Design review of the part built by this model. Coordinates are the model's own, in mm. A direction names the side the tool comes from. Give positions to 0.01 mm unless a question says otherwise; leave off trailing zeros. Loops run counter-clockwise (first coordinate to the right, second up) from the corner with the lowest first, then second, coordinate; pieces in that order, holes last. Notation, with made-up numbers: (-20.5, 74.25) -> (-9.5, 74.25) arc R20 cw to (-9.5, 101.25) -> close; hole circle Ø2 at (8.5, 58). An arc over 180 degrees is marked (long way). Use CSV: the item, a comma, the result in double quotes. Start each with the question number.
Item 1: We need section A-A (x = 6.5). State the section outline as (y, z) points.
Item 2: Clearance check with flat-ended pins moving along their axes: pin 1 (4.5 mm diameter, centred on x = 5, y = 23, fed in from +Z); pin 2 (1.7 mm diameter, centred on x = 6, y = 22.5, fed in from -Z); pin 3 (1 mm diameter, centred on x = 9.5, z = -1.5, fed in from +Y). State where each tip first meets the part, or that it passes through.
Item 3: The part is to be moulded in two halves that separate along Z. For faces 1 (the face through (5.4, 18.4, -1.8)), 2 (the face through (6, 18, -5.6)), 3 (the face through (9.24, 21.85, -2.43)), 4 (the face through (5, 23, -3.89)), say which applies: +Z half, -Z half, draft (parallel to the pull), parting line (faces both ways), or undercut.
Item 4: We need section C-C (z = -5.25). State the section outline as (x, y) points, plus the area to 3 significant figures.
Item 5: Wall thickness on line 1 along Z through (x, y) = (3.25, 6); line 2 along Z through (x, y) = (3.75, 3); line 3 along Z through (x, y) = (7.25, 22): over which ranges is each line inside the solid? List them lowest first. Write a range as from..to.
Item 6: For faces 5 (the face through (9.4, 17.89, -4.91)), 6 (the face through (5, 17.4, -6)), 7 (the face through (6, 5, -2.75)), list the 3-axis set-ups (+Z, -Z, +X, -X, +Y, -Y) from which the entire face can be reached by the end or side of a thin tool; tool diameter is ignored.
Item 7: We need section D-D (y = 24). State the section outline as (x, z) points (3 decimals), plus the area to 3 significant figures.
from build123d import *

# Parameters (mm, degrees)
BOSS_EXTRUDE1_DEPTH = 17.4
BOSS_EXTRUDE2_DEPTH = 1
BOSS_EXTRUDE3_DEPTH = 7
CUT_EXTRUDE1_DEPTH  = 4
CUT_EXTRUDE2_DEPTH  = 6.5
BOSS_EXTRUDE4_DEPTH = 2.1


with BuildPart() as part:
    # Sketch1 → Boss-Extrude1 (new body)
    with BuildSketch(Plane(origin=(0, 0, 0), x_dir=(1, 0, 0), z_dir=(0, 1, 0))):
        with BuildLine():
            Line((3.29, 0), (7.71, 0))
            ThreePointArc((7.71, 0), (10.03638131, 0.96361869), (11, 3.29))
            Line((11, 3.29), (11, 3.31))
            ThreePointArc((11, 3.31), (10.03638131, 5.63638131), (7.71, 6.6))
            Line((7.71, 6.6), (3.29, 6.6))
            ThreePointArc((3.29, 6.6), (0.96361869, 5.63638131), (0, 3.31))
            Line((0, 3.31), (0, 3.29))
            ThreePointArc((0, 3.29), (0.96361869, 0.96361869), (3.29, 0))
        make_face()
    extrude(amount=BOSS_EXTRUDE1_DEPTH)

    # Sketch2 → Boss-Extrude2 (add)
    with BuildSketch(Plane(origin=(0, 17.4, 0), x_dir=(1, 0, 0), z_dir=(0, 1, 0))):
        with BuildLine():
            Line((3.24, 1), (7.76, 1))
            ThreePointArc((7.76, 1), (9.379274529, 1.670725471), (10.05, 3.29))
            Line((10.05, 3.29), (10.05, 3.31))
            ThreePointArc((10.05, 3.31), (9.379274529, 4.929274529), (7.76, 5.6))
            Line((7.76, 5.6), (3.24, 5.6))
            ThreePointArc((3.24, 5.6), (1.620725471, 4.929274529), (0.95, 3.31))
            Line((0.95, 3.31), (0.95, 3.29))
            ThreePointArc((0.95, 3.29), (1.620725471, 1.670725471), (3.24, 1))
        make_face()
    extrude(amount=BOSS_EXTRUDE2_DEPTH)

    # Sketch3 → Boss-Extrude3 (add)
    with BuildSketch(Plane(origin=(0, 18.4, 0), x_dir=(1, 0, 0), z_dir=(0, 1, 0))):
        with BuildLine():
            Line((2.59, 2.09), (8.41, 2.09))
            ThreePointArc((8.41, 2.09), (9.25145707, 2.43854293), (9.6, 3.28))
            Line((9.6, 3.28), (9.6, 3.3))
            ThreePointArc((9.6, 3.3), (9.25145707, 4.14145707), (8.41, 4.49))
            Line((8.41, 4.49), (2.59, 4.49))
            ThreePointArc((2.59, 4.49), (1.74854293, 4.14145707), (1.4, 3.3))
            Line((1.4, 3.3), (1.4, 3.28))
            ThreePointArc((1.4, 3.28), (1.74854293, 2.43854293), (2.59, 2.09))
        make_face()
    extrude(amount=BOSS_EXTRUDE3_DEPTH)

    # Sketch4 → Cut-Extrude1 (cut)
    with BuildSketch(Plane(origin=(0, 25.4, 0), x_dir=(1, 0, 0), z_dir=(0, 1, 0))):
        with BuildLine():
            Line((2.59, 3.89), (8.41, 3.89))
            ThreePointArc((8.41, 3.89), (8.828957038, 3.715421473), (8.999978813, 3.295))
            ThreePointArc((8.999978813, 3.295), (8.832522189, 2.868133654), (8.41, 2.69))
            Line((8.41, 2.69), (2.59, 2.69))
            ThreePointArc((2.59, 2.69), (2.171042962, 2.864578527), (2.000021187, 3.285))
            ThreePointArc((2.000021187, 3.285), (2.167477811, 3.711866346), (2.59, 3.89))
        make_face()
    extrude(amount=-CUT_EXTRUDE1_DEPTH, mode=Mode.SUBTRACT)

    # Sketch5 → Cut-Extrude2 (cut)
    with BuildSketch(Plane.XZ):
        with BuildLine():
            Line((2.55, -4.75), (8.45, -4.75))
            ThreePointArc((8.45, -4.75), (9.298528137, -4.398528137), (9.65, -3.55))
            Line((9.65, -3.55), (9.65, -3.05))
            ThreePointArc((9.65, -3.05), (9.298528137, -2.201471863), (8.45, -1.85))
            Line((8.45, -1.85), (2.55, -1.85))
            ThreePointArc((2.55, -1.85), (1.701471863, -2.201471863), (1.35, -3.05))
            Line((1.35, -3.05), (1.35, -3.55))
            ThreePointArc((1.35, -3.55), (1.701471863, -4.398528137), (2.55, -4.75))
        make_face()
    extrude(amount=-CUT_EXTRUDE2_DEPTH, mode=Mode.SUBTRACT)

    # Sketch6 → Boss-Extrude4 (add)
    with BuildSketch(Plane.XZ.offset(-6.5)):
        with BuildLine():
            Line((2.59, -3.85), (8.41, -3.85))
            ThreePointArc((8.41, -3.85), (8.791837662, -3.691837662), (8.95, -3.31))
            Line((8.95, -3.31), (8.95, -3.29))
            ThreePointArc((8.95, -3.29), (8.791837662, -2.908162338), (8.41, -2.75))
            Line((8.41, -2.75), (2.59, -2.75))
            ThreePointArc((2.59, -2.75), (2.208162338, -2.908162338), (2.05, -3.29))
            Line((2.05, -3.29), (2.05, -3.31))
            ThreePointArc((2.05, -3.31), (2.208162338, -3.691837662), (2.59, -3.85))
        make_face()
    extrude(amount=BOSS_EXTRUDE4_DEPTH)


solid = part.part
Results found:
1,outline,"(0, -6.6) -> (17.4, -6.6) -> (17.4, -5.6) -> (18.4, -5.6) -> (18.4, -4.49) -> (25.4, -4.49) -> (25.4, -3.89) -> (21.4, -3.89) -> (21.4, -2.69) -> (25.4, -2.69) -> (25.4, -2.09) -> (18.4, -2.09) -> (18.4, -1) -> (17.4, -1) -> (17.4, 0) -> (0, 0) -> (0, -1.85) -> (6.5, -1.85) -> (6.5, -2.75) -> (4.4, -2.75) -> (4.4, -3.85) -> (6.5, -3.85) -> (6.5, -4.75) -> (0, -4.75) -> close"
2,pin 1,"z = -2.09"
2,pin 2,"z = -4.49"
2,pin 3,"y = 18.4"
3,face 1,"draft"
3,face 2,"-Z half"
3,face 3,"+Z half"
3,face 4,"undercut"
4,outline,"(0.63, 0) -> (10.37, 0) -> (10.37, 17.4) -> (8.98, 17.4) -> (8.98, 18.4) -> (2.02, 18.4) -> (2.02, 17.4) -> (0.63, 17.4) -> close"
4,area,"176 mm²"
5,line 1,"-6.6..-4.75, -3.85..-2.75, -1.85..0"
5,line 2,"-6.6..-4.75, -1.85..0"
5,line 3,"-4.49..-3.89, -2.69..-2.09"
6,face 5,"-Z, +X, +Y"
6,face 6,"+Y"
6,face 7,"-Y"
7,outline,"(1.4, -3.3) arc R1.19 ccw to (2.59, -4.49) -> (8.41, -4.49) arc R1.19 ccw to (9.6, -3.3) -> (9.6, -3.28) arc R1.19 ccw to (8.41, -2.09) -> (2.59, -2.09) arc R1.19 ccw to (1.4, -3.28) -> close; hole (2, -3.285) arc R0.59 ccw to (2.59, -3.89) -> (8.41, -3.89) arc R0.59 ccw to (9, -3.295) arc R0.59 ccw to (8.41, -2.69) -> (2.59, -2.69) arc R0.59 ccw to start"
7,area,"10.4 mm²"
